Source: three-view drawing plus pictorial views. Frame: mm from the lowest corner of the part. A direction names the side the tool comes from. Round coordinates to 2 decimals unless told otherwise and drop trailing zeros. Loops run counter-clockwise (first coordinate to the right, second up) from the corner with the lowest first, then second, coordinate; pieces in that order, holes last. Notation, with made-up numbers: (17.25, 69.5) -> (63.25, 69.5) arc R9 cw to (63.25, 80.5) -> close; hole circle Ø10 at (-34.5, 57). An arc over 180 degrees is marked (long way). Put each result on its own line as item: value. Start each with the question number.
1. Material intervals for L1, parallel to X at y = 114.3, z = 0.95; L2, parallel to X at y = 40, z = 9.25, sorted ascending.
2. Set-up query: the marked faces 1 and 2. Return all of +Z, -Z, +X, -X, +Y, -Y with unobstructed straight access to the full face (end or side cutting, diameter ignored); none if empty.
3. Contact query for flat-ended pins moving along their axis: pin 1 (4 mm diameter, centred on y = 30, z = 10, fed in from -X); pin 2 (2.5 mm diameter, centred on x = 12.7, y = 105.32, fed in from +Z); pin 3 (5 mm diameter, centred on y = 31.75, z = 12.7, fed in from +X). Output: stop coordinate, or through.
4. Cut plane A-A (x = 12.7). Return the cut outline in (y, z).
5. Cut plane B-B (z = 12.7). Return the cut outline in (x, y) (1 decimal).
6. Cut plane D-D (y = 31.75). Return the cut outline in (x, z) (1 decimal).
7. Cut plane C-C (y = 114.3). Return the cut outline in (x, z).
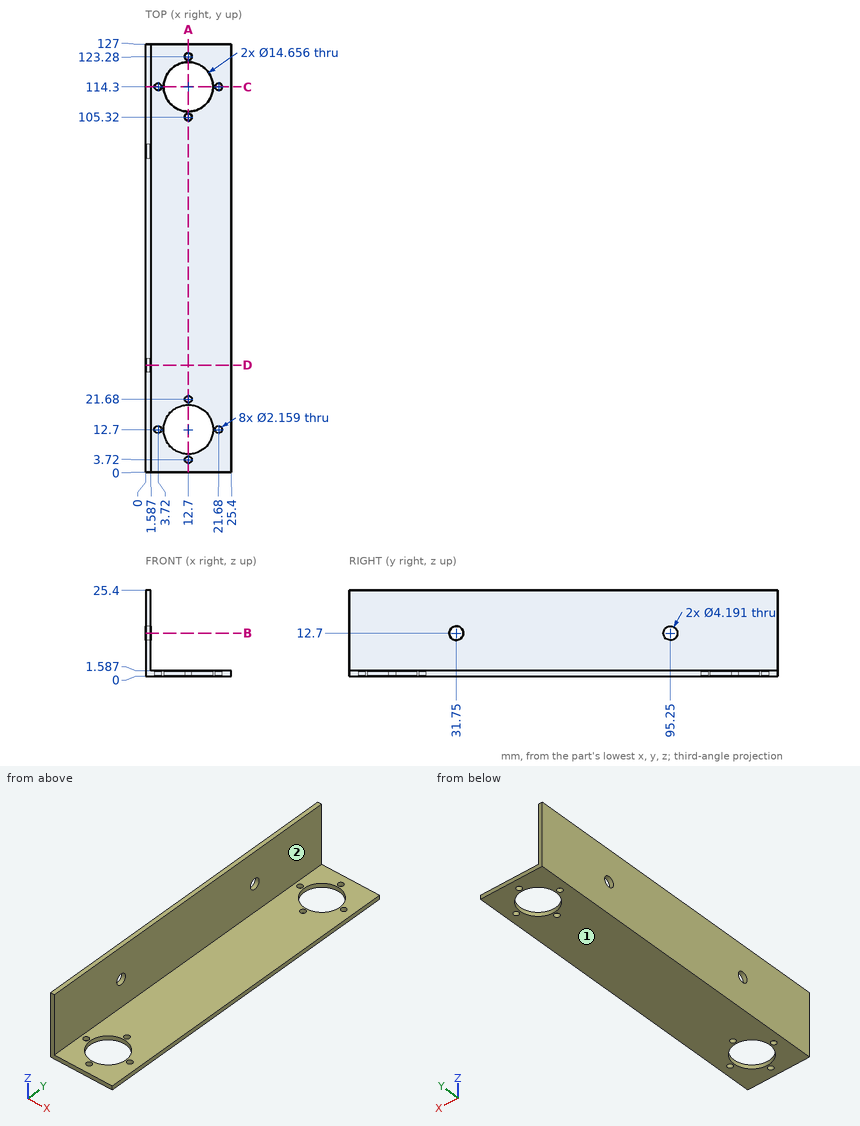
Solution:
1. L1: x = 0 to 2.64, 4.8 to 5.37, 20.03 to 20.6, 22.76 to 25.4
1. L2: x = 0 to 1.59
2. face 1: -Z, +X, -X, +Y, -Y
2. face 2: +Z, +X, +Y, -Y
3. pin 1: stops at x = 0
3. pin 2: stops at z = 1.59
3. pin 3: stops at x = 1.59
4. outline: (0, 0) -> (2.64, 0) -> (2.64, 1.59) -> (0, 1.59) -> close; (4.8, 0) -> (5.37, 0) -> (5.37, 1.59) -> (4.8, 1.59) -> close; (20.03, 0) -> (20.6, 0) -> (20.6, 1.59) -> (20.03, 1.59) -> close; (22.76, 0) -> (104.24, 0) -> (104.24, 1.59) -> (22.76, 1.59) -> close; (106.4, 0) -> (106.97, 0) -> (106.97, 1.59) -> (106.4, 1.59) -> close; (121.63, 0) -> (122.2, 0) -> (122.2, 1.59) -> (121.63, 1.59) -> close; (124.36, 0) -> (127, 0) -> (127, 1.59) -> (124.36, 1.59) -> close
5. outline: (0, 0) -> (1.6, 0) -> (1.6, 29.7) -> (0, 29.7) -> close; (0, 33.8) -> (1.6, 33.8) -> (1.6, 93.2) -> (0, 93.2) -> close; (0, 97.3) -> (1.6, 97.3) -> (1.6, 127) -> (0, 127) -> close
6. outline: (0, 0) -> (25.4, 0) -> (25.4, 1.6) -> (1.6, 1.6) -> (1.6, 10.6) -> (0, 10.6) -> close; (0, 14.8) -> (1.6, 14.8) -> (1.6, 25.4) -> (0, 25.4) -> close
7. outline: (0, 0) -> (2.64, 0) -> (2.64, 1.59) -> (1.59, 1.59) -> (1.59, 25.4) -> (0, 25.4) -> close; (4.8, 0) -> (5.37, 0) -> (5.37, 1.59) -> (4.8, 1.59) -> close; (20.03, 0) -> (20.6, 0) -> (20.6, 1.59) -> (20.03, 1.59) -> close; (22.76, 0) -> (25.4, 0) -> (25.4, 1.59) -> (22.76, 1.59) -> close
